Design review of the part built by this model. Coordinates are the model's own, in mm. A direction names the side the tool comes from. Coordinates: 2 decimals unless noted, no trailing zeros. Loops run counter-clockwise (first coordinate to the right, second up) from the corner with the lowest first, then second, coordinate; pieces in that order, holes last. Notation, with made-up numbers: M 31,58.5 L 75,58.5 A19 ccw 75,91.5 Z; hole C 18,37.25 d6. An arc over 180 degrees is marked long. Write item = value, one per line. Start each with the question number.
from build123d import *

# Parameters (mm, degrees)
SKETCH_1_R      = 71
SKETCH_1_R_2    = 68
EXTRUDE_1_DEPTH = 118
EXTRUDE_START   = 66.5
EXTRUDE_9_DEPTH = 16.5


with BuildPart() as part:
    # 草圖1 → 填料-伸長1 (new body)
    with BuildSketch(Plane(origin=(0, 0, 0), x_dir=(1, 0, 0), z_dir=(0, 1, 0))):
        with Locations(Location((0, 0, 0), (0, 0, 270))):
            Circle(SKETCH_1_R)
        with Locations(Location((0, 0, 0), (0, 0, 270))):
            Circle(SKETCH_1_R_2, mode=Mode.SUBTRACT)
    extrude(amount=EXTRUDE_1_DEPTH)

    # 草圖5 → 填料-伸長9 (add)
    with BuildSketch(Plane(origin=(0, 0, 0), x_dir=(1, 0, 0), z_dir=(0, 1, 0)).offset(EXTRUDE_START)):
        with BuildLine():
            Line((-11, -60.519057708), (-31.007154887, -60.519057708))
            ThreePointArc((-31.007154887, -60.519057708), (0, -68), (31.007154887, -60.519057708))
            Line((31.007154887, -60.519057708), (11, -60.519057708))
            Line((11, -60.519057708), (8.25, -60.519057708))
            Line((8.25, -60.519057708), (-8.25, -60.519057708))
            Line((-8.25, -60.519057708), (-11, -60.519057708))
        make_face()
        with BuildLine():
            ThreePointArc((31.007154887, 60.519057708), (0, 68), (-31.007154887, 60.519057708))
            Line((-31.007154887, 60.519057708), (-11, 60.519057708))
            Line((-11, 60.519057708), (-8.25, 60.519057708))
            Line((-8.25, 60.519057708), (8.25, 60.519057708))
            Line((8.25, 60.519057708), (11, 60.519057708))
            Line((11, 60.519057708), (31.007154887, 60.519057708))
        make_face()
        with BuildLine():
            Line((-60.519057708, -31.007154887), (-60.519057708, -11))
            Line((-60.519057708, -11), (-60.519057708, -8.25))
            Line((-60.519057708, -8.25), (-60.519057708, 8.25))
            Line((-60.519057708, 8.25), (-60.519057708, 11))
            Line((-60.519057708, 11), (-60.519057708, 31.007154887))
            ThreePointArc((-60.519057708, 31.007154887), (-68, 0), (-60.519057708, -31.007154887))
        make_face()
        with BuildLine():
            Line((60.519057708, -11), (60.519057708, -31.007154887))
            ThreePointArc((60.519057708, -31.007154887), (66.103312792, -15.948418039), (68, 0))
            ThreePointArc((68, 0), (66.103312792, 15.948418039), (60.519057708, 31.007154887))
            Line((60.519057708, 31.007154887), (60.519057708, 11))
            Line((60.519057708, 11), (60.519057708, 8.25))
            Line((60.519057708, 8.25), (60.519057708, -8.25))
            Line((60.519057708, -8.25), (60.519057708, -11))
        make_face()
    extrude(amount=EXTRUDE_9_DEPTH)


solid = part.part
Q1. Add section D-D on z = -33. State the section outline as (x, y) points.
Q2. Add section A-A on y = 75.5. State the section outline as (x, z) points, plus the area to 3 significant figures.
Q3. Mouldability with a two-part tool opening along Z and no side actions: class faces 4 (the face through (-63, 83, 0)), 5 (the face through (-36, 0, 58)), 6 (the face through (-62.99, 58.17, 32.76)) as released by +Z, released by -Z, zero draft, split by the parting line, or undercut.
Q4. Clearance check with flat-ended pins moving along their axes: P1, Ø2, axis at x = 64.5, z = -11.5, coming from the -Y side; P2, Ø8, axis at x = -33, y = 85.5, coming from the +Z side; P3, Ø18, axis at x = -14, y = 72.5, coming from the -Z side. State where each tip first meets the part, or that it passes through.
Q5. Add section C-C on z = 0. State the section outline as (x, y) points.
Q6. To check wall thickness, follow line 1 (X direction, y = 41.5, z = 0); line 2 (X direction, y = 69, z = 1); line 3 (Z direction, x = 42.5, y = 49). State the ranges of each line that lie inside material, in increasing order. Write a range as from..to.
Q7. For faces 1 (the face through (0, 66.5, 63)), 2 (the face through (0, 75, -60.519)), 3 (the face through (2.99, 58.174, -67.934)), list the 3-axis set-ups (+Z, -Z, +X, -X, +Y, -Y) from which the entire face can be reached by the end or side of a thin tool; tool diameter is ignored.
Q8. Add section B-B on x = 0. State the section outline as (y, z) points.
Values follow:
q1.outline = M -62.86,0 L -59.46,0 L -59.46,118 L -62.86,118 Z; M 59.46,0 L 62.86,0 L 62.86,118 L 59.46,118 Z
q2.outline = C 0,0 d142; hole M -60.52,-31.01 A68 ccw -31.01,-60.52 L 31.01,-60.52 A68 ccw 60.52,-31.01 L 60.52,31.01 A68 ccw 31.01,60.52 L -31.01,60.52 A68 ccw -60.52,31.01 Z
q2.area = 2,560 mm2
q3.face_4 = undercut
q3.face_5 = zero draft
q3.face_6 = split by the parting line
q4.P1 = 66.5
q4.P2 = 64.81
q4.P3 = -70.82
q5.outline = M -71,0 L -68,0 L -68,66.5 L -60.52,66.5 L -60.52,83 L -68,83 L -68,118 L -71,118 Z; M 60.52,66.5 L 68,66.5 L 68,0 L 71,0 L 71,118 L 68,118 L 68,83 L 60.52,83 Z
q6.line_1 = -71..-68, 68..71
q6.line_2 = -70.99..-60.52, 60.52..70.99
q6.line_3 = -56.87..-53.08, 53.08..56.87
q7.face_1 = -Y
q7.face_2 = +Y, -Y
q7.face_3 = none
q8.outline = M 0,-71 L 118,-71 L 118,-68 L 83,-68 L 83,-60.52 L 66.5,-60.52 L 66.5,-68 L 0,-68 Z; M 0,68 L 66.5,68 L 66.5,60.52 L 83,60.52 L 83,68 L 118,68 L 118,71 L 0,71 Z
